Work out the finished part from the listing and answer in its coordinate system (mm). A direction names the side the tool comes from. Give positions to 0.01 mm unless a question says otherwise; leave off trailing zeros. Loops run counter-clockwise (first coordinate to the right, second up) from the corner with the lowest first, then second, coordinate; pieces in that order, holes last. Notation, with made-up numbers: M -12,-22 L 8,-22 A19 cw 8,4 Z; hole C 74.25,10 d3. An arc over 180 degrees is marked long. Answer as a JSON object with one key per item and string values. Group by question number.
Autodesk Fusion 360 part; units mm, degrees
sketch "Sketch3" plane through (0, 0, 0) normal (1, 0, 0) x (0, 1, 0)
  line L0 (0, 0) -> (28.7888, 0)
  line L1 (28.7888, 0) -> (28.7888, 106.2286)
  line L2 (28.7888, 106.2286) -> (8.923, 106.2286)
  line L3 (8.923, 106.2286) -> (8.923, 142.7466)
  line L4 (6.2937, 142.7466) -> (6.2937, 100.0936)
  line L5 (6.2937, 100.0936) -> (26.1595, 100.0936)
  line L6 (26.1595, 100.0936) -> (26.1595, 3.6859)
  line L7 (26.1595, 3.6859) -> (0, 3.6859)
  line L8 (0, 3.6859) -> (0, 0)
  line L9 (8.923, 142.7466) -> (6.2937, 142.7466)
revolve "Revolve2" add sketch "Sketch3" angle 360 about axis through (0, 0, 1.75) along (0, 0, 1)
fillet "Fillet10" radius 10 1 edges at (-26.8406, 10.4105, 106.2286)
fillet "Fillet11" radius 10 1 edges at (-8.3191, 3.2267, 106.2286)
fillet "Fillet12" radius 1 1 edges at (-8.3191, 3.2267, 142.7466)
fillet "Fillet13" radius 5 1 edges at (-26.8406, 10.4105, 0)
Item 1: For a pull along X with two mould halves and no side action, classify faces 1 (the cylindrical face through (5.31, 3.38, 121.12)), 2 (the flat face through (0, 0, 0)), 3 (the cylindrical face through (-8.847, -1.162, 129.166)) as pulls with the +X half, pulls with the -X half, needs draft (parallel to the pull), parting line crosses it, or undercut.
Item 2: A tool of negligible diameter and unlimited length cuts with its end or side. For faces 4 (the cylindrical face through (-25.537, -5.671, 51.215)), 5 (the cylindrical face through (28.104, -6.241, 51.253)), from which of +Z, -Z, +X, -X, +Y, -Y can it reach the whole face along a straight path? Write none if from no direction.
Item 3: Given pin 1 Ø10 at (y, z) = (15, 39) entering from +X; pin 2 Ø1.5 at (x, y) = (-10, -5.5) entering from +Z; pin 3 Ø6 at (y, z) = (10.5, 20) entering from +X, each flat-ended and moving along its own axis, determine where each tip first touches the part or whether it passes through.
Item 4: Find the intervals of material crossed by probe 1 along Z at (x, y) = (-1.5, 18.5); probe 2 along X at (y, z) = (0, 68), in increasing order. Write a range as [from, to].
Item 5: A cutting plane is placed at A-A (z = 71.5). Determine the outline of the cut face in (x, y), and give its area (3 significant figures).
Item 6: A cutting plane is placed at B-B (z = 128). Determine the outline of the cut face in (x, y).
The answers:
{
 "1": {"face 1": "undercut", "face 2": "needs draft", "face 3": "parting line crosses it"},
 "2": {"face 4": "none", "face 5": "+Z, -Z"},
 "3": {"pin 1": "stops at x = 27", "pin 2": "stops at z = 110.59", "pin 3": "stops at x = 27.79"},
 "4": {"probe 1": "z = [0, 3.69], [100.09, 106.23]", "probe 2": "x = [-28.79, -26.16], [26.16, 28.79]"},
 "5": {"outline": "C 0,0 d57.58; hole C 0,0 d52.32", "area": "454 mm^2"},
 "6": {"outline": "C 0,0 d17.85; hole C 0,0 d12.59"}
}
